Job drawing, mm, ordinate dimensions from the low corner. One solid piece. Round coordinates to 2 decimals unless told otherwise and drop trailing zeros. Loops run counter-clockwise (first coordinate to the right, second up) from the corner with the lowest first, then second, coordinate; pieces in that order, holes last. Notation, with made-up numbers: M 31.5,-16.5 L 42.5,-16.5 A14 ccw 42.5,-12.5 Z; hole C -19.5,64.5 d1. An arc over 180 degrees is marked long. Use one line per item in the form item = value. Start each with the question number.
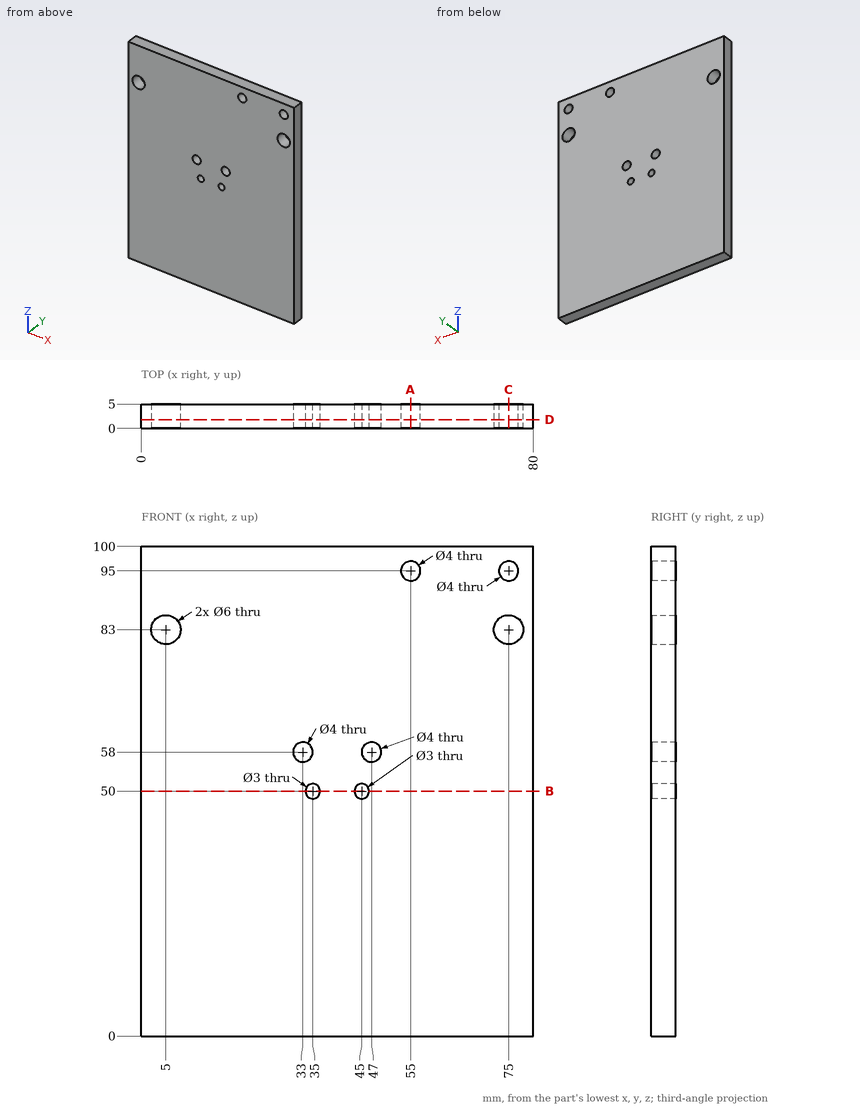
Q1. Wall check: probe 1 along X at (y, z) = (4.55, 56.5); probe 2 along Z at (x, y) = (55, 2.7); probe 3 along Z at (x, y) = (33, 1.55). Give the ranges that are in metal, low to high.
Q2. Saw through at D-D (y = 1.8). Give the number of separate pieces and of enclosed holes in the cut face, and give its area (3 significant figures).
Q3. Saw through at C-C (x = 75). Give the cut face in (y, z).
Q4. Drop flat-ended pins along their axis: P1, Ø3, axis at x = 75, z = 95, coming from the -Y side; P2, Ø8, axis at x = 75, z = 83, coming from the +Y side. Give the stop position or say it passes through.
Q5. Saw through at B-B (z = 50). Give the cut face in (x, y), and give its area (3 significant figures).
Q6. Saw through at A-A (x = 55). Give the cut face in (y, z), and give its area (3 significant figures).
Filled in:
q1.probe_1 = 0 to 31.68, 34.32 to 45.68, 48.32 to 80
q1.probe_2 = 0 to 93, 97 to 100
q1.probe_3 = 0 to 56, 60 to 100
q2.separate_pieces = 1
q2.enclosed_holes = 8
q2.area = 7,880 mm²
q3.outline = M 0,0 L 5,0 L 5,80 L 0,80 Z; M 0,86 L 5,86 L 5,93 L 0,93 Z; M 0,97 L 5,97 L 5,100 L 0,100 Z
q4.P1 = through
q4.P2 = 5
q5.outline = M 0,0 L 33.5,0 L 33.5,5 L 0,5 Z; M 36.5,0 L 43.5,0 L 43.5,5 L 36.5,5 Z; M 46.5,0 L 80,0 L 80,5 L 46.5,5 Z
q5.area = 370 mm²
q6.outline = M 0,0 L 5,0 L 5,93 L 0,93 Z; M 0,97 L 5,97 L 5,100 L 0,100 Z
q6.area = 480 mm²
